from build123d import *

# Parameters (mm, degrees)
EXTRUDE_1_DEPTH     = 30
SKETCH_2_R          = 1.5
CUT_EXTRUDE_1_DEPTH = 20


with BuildPart() as part:
    # 草图1 → 凸台-拉伸1 (new body)
    with BuildSketch(Plane(origin=(0, 0, 0), x_dir=(0, 0, -1), z_dir=(1, 0, 0))):
        Polygon((0, 25), (0, 0), (15, 0), (15, -5), (-5, -5), (-5, 25), align=None)
    extrude(amount=EXTRUDE_1_DEPTH)

    # 草图2 → 切除-拉伸1 (cut)
    with BuildSketch(Plane(origin=(0, 0, 0), x_dir=(1, 0, 0), z_dir=(0, 1, 0))):
        with Locations(Location((5, 5, 0), (0, 0, 270))):
            Circle(SKETCH_2_R)
        with Locations(Location((25, 5, 0), (0, 0, 270))):
            Circle(SKETCH_2_R)
    extrude(amount=-CUT_EXTRUDE_1_DEPTH, mode=Mode.SUBTRACT)


solid = part.part
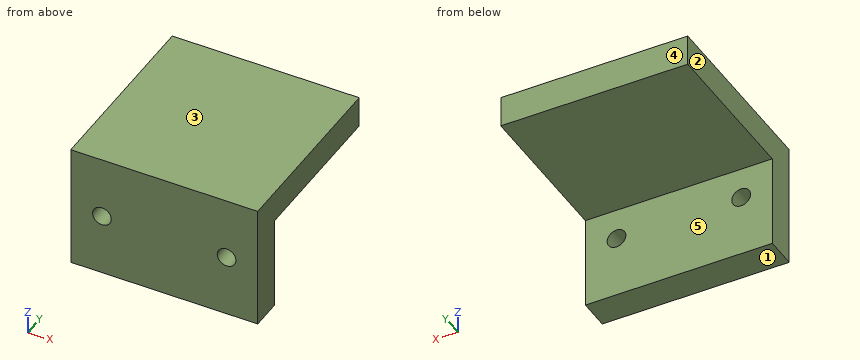
Input: part model. Units: mm. Frame: model coordinates. Face numbers are marked on the shaded views. A direction names the side the tool comes from. Coordinates: 2 decimals unless noted, no trailing zeros. Write each loop counter-clockwise with the first axis right and the second up, starting at its lowest first coordinate (ties: lowest second). Pieces come first, ordered by that corner, then holes. Notation, with made-up numbers: M 72.5,62.25 L 108.5,62.25 A19 cw 108.5,91.25 Z; hole C 47.5,-10 d2. An arc over 180 degrees is marked long. Answer as a JSON object with one key per item and string values. Group by question number.
(1) Section D-D on x = 18.5. Output: boundary loops of the cut face in (y, z), plus the area to 3 significant figures.
(2) Section A-A on z = -5. Output: boundary loops of the cut face in (x, y), plus the area to 3 significant figures.
(3) Section C-C on y = -2. Output: boundary loops of the cut face in (x, z).
(4) Mould query, pull axis Z, two halves, no side actions, for the marked faces 1, 2 and 3. Classes: pulls with the +Z half, pulls with the -Z half, needs draft (parallel to the pull), parting line crosses it, or undercut.
(5) Ray query, line 1 along X through (y, z) = (-2.25, -5); line 2 along Y through (x, z) = (7.5, -0.5); line 3 along Z through (x, y) = (17, 12). Return the intervals inside material, ascending. Write a range as [from, to].
(6) Set-up query: the marked faces 4 and 5. Return all of +Z, -Z, +X, -X, +Y, -Y with unobstructed straight access to the full face (end or side cutting, diameter ignored); none if empty.
(7) Contact query for flat-ended pins moving along their axis: P1, Ø4.5, axis at x = 10, z = -4, coming from the +Y side; P2, Ø1.5, axis at x = 21, y = 12, coming from the -Z side. Output: stop coordinate, or through.
(8) Section B-B on x = 25. Output: boundary loops of the cut face in (y, z).
Result set:
{
 "1": {"outline": "M -5,-15 L 0,-15 L 0,0 L 25,0 L 25,5 L -5,5 Z", "area": "225 mm2"},
 "2": {"outline": "M 0,-5 L 3.5,-5 L 3.5,0 L 0,0 Z; M 6.5,-5 L 23.5,-5 L 23.5,0 L 6.5,0 Z; M 26.5,-5 L 30,-5 L 30,0 L 26.5,0 Z", "area": "120 mm2"},
 "3": {"outline": "M 0,-15 L 30,-15 L 30,5 L 0,5 Z; hole C 5,-5 d3; hole C 25,-5 d3"},
 "4": {"face 1": "pulls with the -Z half", "face 2": "needs draft", "face 3": "pulls with the +Z half"},
 "5": {"line 1": "x = [0, 3.5], [6.5, 23.5], [26.5, 30]", "line 2": "y = [-5, 0]", "line 3": "z = [0, 5]"},
 "6": {"face 4": "+Z, -Z, +X, -X, +Y", "face 5": "-Z, +X, -X, +Y"},
 "7": {"P1": "stops at y = 0", "P2": "stops at z = 0"},
 "8": {"outline": "M -5,-15 L 0,-15 L 0,-6.5 L -5,-6.5 Z; M -5,-3.5 L 0,-3.5 L 0,0 L 25,0 L 25,5 L -5,5 Z"}
}
